Build history of the part. All positions in model axes, mm. Round coordinates to 2 decimals unless told otherwise and drop trailing zeros.
from build123d import *

# Parameters (mm, degrees)
F2_DEPTH     = 6.35
F3_T6_ANGLE  = 79.5586583167
F3_T8_ANGLE  = 79.5586583167
F3_T10_ANGLE = 63.5249338853
F3_T12_ANGLE = 63.5249338853
F3_T14_ANGLE = 109.1774772549
F3_T16_ANGLE = 109.1774772549
F3_T18_ANGLE = 50.5483837844
F3_T20_ANGLE = 50.5483837844


# Not quite as in the source:
# - a fillet or chamfer that OpenCascade refuses, or shapes differently, is made with other operations: its cross-section is extruded or revolved along the edge and cut away or added


with BuildPart() as f2:
    # F1 (on Top) → F2 (new body)
    with BuildSketch(Plane.XY):
        with BuildLine():
            ThreePointArc((-73.1568782646, -21.3192674026), (-75.6518657205, 9.1233334372), (-65.9911357684, 38.1))
            ThreePointArc((-65.9911357684, 38.1), (-73.5398929218, 37.7251690762), (-81.0143847835, 36.6043639223))
            ThreePointArc((-81.0143847835, 36.6043639223), (-88.9, 0), (-81.0143847835, -36.6043639223))
            ThreePointArc((-81.0143847835, -36.6043639223), (-73.8686107341, -39.0834183952), (-66.5806584514, -37.0601662189))
            ThreePointArc((-66.5806584514, -37.0601662189), (-68.3796387065, -33.6253626057), (-70.0015683829, -30.1034952113))
            ThreePointArc((-70.0015683829, -30.1034952113), (-78.2486807064, -28.1070619795), (-73.1568782646, -21.3192674026))
        make_face()
        with BuildLine():
            ThreePointArc((0, 0), (-27.8911357684, 27.8911357684), (-65.9911357684, 38.1))
            ThreePointArc((-65.9911357684, 38.1), (-75.6518657205, 9.1233334372), (-73.1568782646, -21.3192674026))
            ThreePointArc((-73.1568782646, -21.3192674026), (-69.7673746876, -22.9092911449), (-68.3877575616, -26.3897460844))
            ThreePointArc((-68.3877575616, -26.3897460844), (-68.8086460032, -28.4143644401), (-70.0015683829, -30.1034952113))
            ThreePointArc((-70.0015683829, -30.1034952113), (-68.3796387065, -33.6253626057), (-66.5806584514, -37.0601662189))
            ThreePointArc((-66.5806584514, -37.0601662189), (-65.2319724125, -36.0573126333), (-64.0275195551, -34.8851511001))
            ThreePointArc((-64.0275195551, -34.8851511001), (-63.0707476834, -33.4387934378), (-62.0813092162, -32.0145833333))
            ThreePointArc((-62.0813092162, -32.0145833333), (-34.925, -8.4749354005), (0, 0))
        make_face()
    extrude(amount=F2_DEPTH)

    # F3: chamfer of 2.1166666667 on 10 edges, made by hand

    # F3_s1 → F3_t2 (revolve, cut)
    with BuildSketch(Plane(origin=(-71.580679249, 4.3887278976, 0), x_dir=(0, 0, 1), z_dir=(-0.9981257248, 0.061196712, 0))):
        Polygon((4.2333333333, -25.7562696385), (6.35, -23.6396029718), (6.35, -25.7562696385), align=None)
    revolve(axis=Axis((-73.4677575616, -26.3897460844, 6.35), (0, 0, -1)), mode=Mode.SUBTRACT)

    # F3_s3 → F3_t4 (revolve, cut)
    with BuildSketch(Plane(origin=(-71.580679249, 4.3887278976, 0), x_dir=(0, 0, 1), z_dir=(-0.9981257248, 0.061196712, 0))):
        Polygon((0, -23.6396029718), (2.1166666667, -25.7562696385), (0, -25.7562696385), align=None)
    revolve(axis=Axis((-73.4677575616, -26.3897460844, 0), (0, 0, -1)), mode=Mode.SUBTRACT)

    # F3_s5 → F3_t6 (revolve, cut)
    with BuildSketch(Plane(origin=(2.3767752158, -4.8934699303, 0), x_dir=(0, 0, 1), z_dir=(0.4368960746, -0.8995119899, 0))):
        Polygon((4.2333333333, -0.1944417058), (6.35, 1.9222249609), (6.35, -0.1944417058), align=None)
    revolve(axis=Axis((-65.9911357684, -38.1, 6.35), (0, 0, 1)), revolution_arc=F3_T6_ANGLE, mode=Mode.SUBTRACT)

    # F3_s7 → F3_t8 (revolve, cut)
    with BuildSketch(Plane(origin=(2.3767752158, -4.8934699303, 0), x_dir=(0, 0, 1), z_dir=(0.4368960746, -0.8995119899, 0))):
        Polygon((0, 1.9222249609), (2.1166666667, -0.1944417058), (0, -0.1944417058), align=None)
    revolve(axis=Axis((-65.9911357684, -38.1, 0), (0, 0, 1)), revolution_arc=F3_T8_ANGLE, mode=Mode.SUBTRACT)

    # F3_s9 → F3_t10 (revolve, cut)
    with BuildSketch(Plane(origin=(-32.1255217702, -58.583184591, 0), x_dir=(0, 0, 1), z_dir=(-0.4808240877, -0.8768170828, 0))):
        Polygon((6.35, 41.6778711875), (4.2333333333, 39.5612045208), (6.35, 39.5612045208), align=None)
    revolve(axis=Axis((0, -76.2, 6.35), (0, 0, -1)), revolution_arc=F3_T10_ANGLE, mode=Mode.SUBTRACT)

    # F3_s11 → F3_t12 (revolve, cut)
    with BuildSketch(Plane(origin=(-32.1255217702, -58.583184591, 0), x_dir=(0, 0, 1), z_dir=(-0.4808240877, -0.8768170828, 0))):
        Polygon((0, 41.6778711875), (2.1166666667, 39.5612045208), (0, 39.5612045208), align=None)
    revolve(axis=Axis((0, -76.2, 0), (0, 0, -1)), revolution_arc=F3_T12_ANGLE, mode=Mode.SUBTRACT)

    # F3_s13 → F3_t14 (revolve, cut)
    with BuildSketch(Plane(origin=(-6.0616572407, 10.9442518524, 0), x_dir=(0, 0, 1), z_dir=(-0.484513618, 0.8747837184, 0))):
        Polygon((4.2333333333, -89.7545894961), (6.35, -87.6379228294), (6.35, -89.7545894961), align=None)
    revolve(axis=Axis((-73.4677575616, -26.3897460844, 6.35), (0, 0, 1)), revolution_arc=F3_T14_ANGLE, mode=Mode.SUBTRACT)

    # F3_s15 → F3_t16 (revolve, cut)
    with BuildSketch(Plane(origin=(-6.0616572407, 10.9442518524, 0), x_dir=(0, 0, 1), z_dir=(-0.484513618, 0.8747837184, 0))):
        Polygon((0, -87.6379228294), (2.1166666667, -89.7545894961), (0, -89.7545894961), align=None)
    revolve(axis=Axis((-73.4677575616, -26.3897460844, 0), (0, 0, 1)), revolution_arc=F3_T16_ANGLE, mode=Mode.SUBTRACT)

    # F3_s17 → F3_t18 (revolve, cut)
    with BuildSketch(Plane(origin=(0, 0, 0), x_dir=(0, 0, 1), z_dir=(0.4407105264, 0.8976492811, 0))):
        Polygon((4.2333333333, -88.9), (6.35, -86.7833333333), (6.35, -88.9), align=None)
    revolve(axis=Axis((0, 0, 6.35), (0, 0, 1)), revolution_arc=F3_T18_ANGLE, mode=Mode.SUBTRACT)

    # F3_s19 → F3_t20 (revolve, cut)
    with BuildSketch(Plane(origin=(0, 0, 0), x_dir=(0, 0, 1), z_dir=(0.4407105264, 0.8976492811, 0))):
        Polygon((2.1166666667, -88.9), (0, -86.7833333333), (0, -88.9), align=None)
    revolve(axis=Axis((0, 0, 0), (0, 0, 1)), revolution_arc=F3_T20_ANGLE, mode=Mode.SUBTRACT)


solid = f2.part
(1) Probe line 1 (Y direction, x = -69, z = 4); line 2 (Y direction, x = -78.5, z = 6); line 3 (X direction, y = -30.5, z = 5.5). List the from-to ranges inside material, lowest first.
Responses:
line 1: y = -38.28 to -28.81, -23.97 to 38.04
line 2: y = -36.1 to -31.03, -21.75 to 35.27
line 3: x = -82.15 to -78.3, -68.63 to -62.55
(2) Pin check, flat tips, straight feed: P1, Ø5, axis at x = -10, y = 9.5, coming from the -Z side; P2, Ø1.5, axis at x = -39, z = 5, coming from the +Y side; P3, Ø1.5, axis at x = -38.5, z = 1, coming from the +Y side. Stop position of each tip, or through.
Responses:
P1: stops at z = 0
P2: stops at y = 33.19
P3: stops at y = 32.63
(3) Pull direction X, two halves, no side cores. Call faces 1 (the face through (-55, 8, 0)), 2 (the face through (-88.9, 0.5, 3.2)), 3 (the face through (-68.351, -27.383, 4.366)): +X half, -X half, draft (parallel to the pull), parting line (faces both ways), or undercut.
Responses:
face 1: draft
face 2: -X half
face 3: undercut
